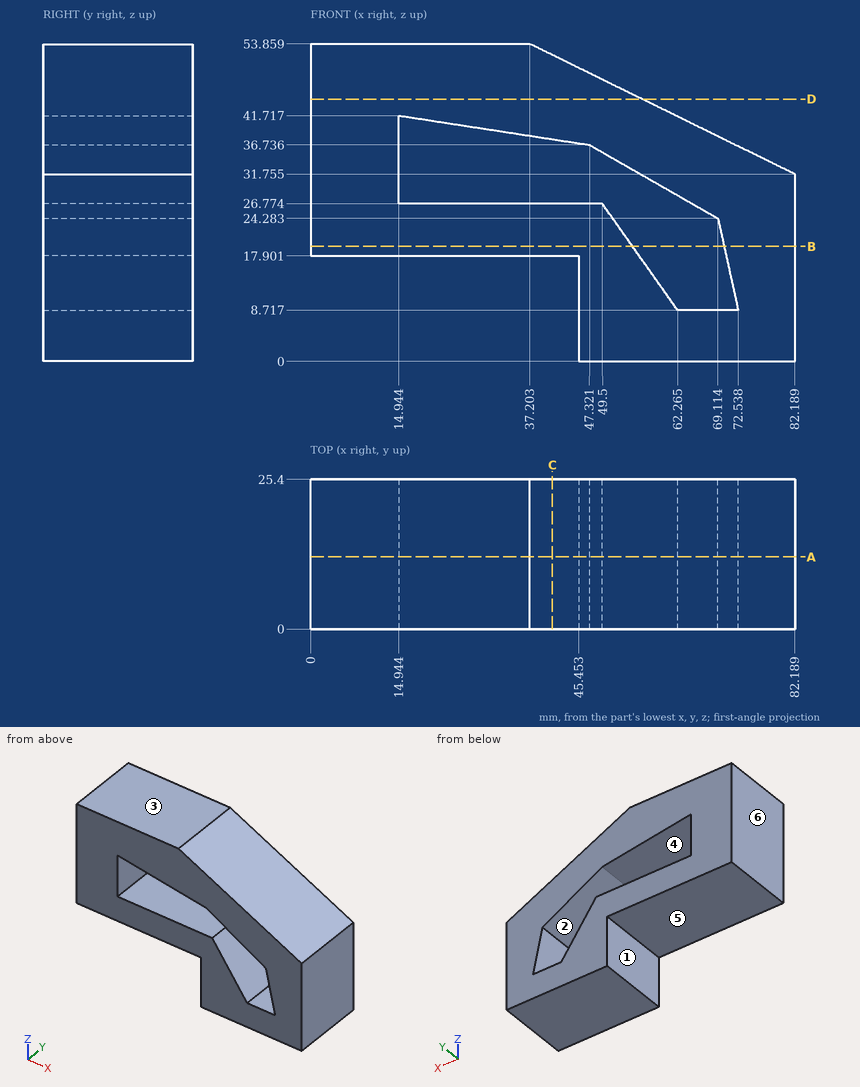
The figure shows three views and two pictorial views of one solid part (mm, origin at its lowest corner). Answer the questions. A direction names the side the tool comes from. Round coordinates to 2 decimals unless told otherwise and drop trailing zeros. Loops run counter-clockwise (first coordinate to the right, second up) from the corner with the lowest first, then second, coordinate; pieces in that order, holes last. Notation, with made-up numbers: M 78,0.25 L 125,0.25 A23 cw 125,13.25 Z; hole C 61.5,-25.75 d4. An arc over 180 degrees is marked long. Return JSON: item names as keys, results as strings.
Q1. Which of the six approach directions +Z, -Z, +X, -X, +Y, -Y give full straight-line access (tool end or side, diameter ignored) to the marked faces 4, 5 and 6?
Results list:
{"face 4": "+Y, -Y", "face 5": "-Z, -X, +Y, -Y", "face 6": "+Z, -Z, -X, +Y, -Y"}
Q2. Find the intervals of material crossed by line 1 along X through (y, z) = (11.25, 22) (1 decimal); line 2 along X through (y, z) = (6.75, 2); line 3 along Z through (x, y) = (34.5, 6) (1 decimal), in increasing order. Write a range as from..to.
Results list:
{"line 1": "x = 0..52.9, 69.6..82.2", "line 2": "x = 45.45..82.19", "line 3": "z = 17.9..26.8, 38.7..53.9"}
Q3. Find section A-A, the plane y = 12.25. Determine the outline of the cut face in (x, z) (1 decimal).
Results list:
{"outline": "M 0,17.9 L 45.5,17.9 L 45.5,0 L 82.2,0 L 82.2,31.8 L 37.2,53.9 L 0,53.9 Z; hole M 14.9,26.8 L 49.5,26.8 L 62.3,8.7 L 72.5,8.7 L 69.1,24.3 L 47.3,36.7 L 14.9,41.7 Z"}
Q4. The mould has two halves that part along X. Classify the marked faces 1, 2 and 3: released by +X, released by -X, zero draft, split by the parting line, or undercut.
Results list:
{"face 1": "released by -X", "face 2": "undercut", "face 3": "zero draft"}
Q5. Find section D-D, the plane z = 44.5. Determine the outline of the cut face in (x, y), plus the area to 3 significant figures.
Results list:
{"outline": "M 0,0 L 56.25,0 L 56.25,25.4 L 0,25.4 Z", "area": "1,430 mm2"}
Q6. Each of these flat-tipped pins is pushed along its axis until it touches: pin 1 Ø5.5 at (y, z) = (11.5, 5.5) entering from -X; pin 2 Ø5 at (x, y) = (67, 9.5) entering from +Z; pin 3 Ø7.5 at (y, z) = (10, 35) entering from +X; pin 4 Ø7.5 at (x, y) = (34, 17) entering from -Z. Where does it stop, or does it pass through?
Results list:
{"pin 1": "stops at x = 45.45", "pin 2": "stops at z = 40.45", "pin 3": "stops at x = 82.19", "pin 4": "stops at z = 17.9"}
Q7. Find section C-C, the plane x = 41. Determine the outline of the cut face in (y, z).
Results list:
{"outline": "M 0,17.9 L 25.4,17.9 L 25.4,26.77 L 0,26.77 Z; M 0,37.71 L 25.4,37.71 L 25.4,51.99 L 0,51.99 Z"}
Q8. Find section B-B, the plane z = 19.5. Determine the outline of the cut face in (x, y) (1 decimal).
Results list:
{"outline": "M 0,0 L 54.6,0 L 54.6,25.4 L 0,25.4 Z; M 70.2,0 L 82.2,0 L 82.2,25.4 L 70.2,25.4 Z"}
